```python
from build123d import *

# Parameters (mm, degrees)
SALIENTE_EXTRUIR1_DEPTH = 13.746
CROQUIS2_R              = 15.5
CORTAR_EXTRUIR1_DEPTH   = 10
CROQUIS3_R              = 1.6
CORTAR_EXTRUIR2_DEPTH   = 10
SALIENTE_EXTRUIR2_START = -4
CROQUIS4_R              = 1.5
SALIENTE_EXTRUIR2_DEPTH = 4
CORTAR_EXTRUIR3_DEPTH   = 45.978374576
CROQUIS6_R              = 1.5
CORTAR_EXTRUIR4_DEPTH   = 44.749194214
CROQUIS7_R              = 2.05
CORTAR_EXTRUIR5_DEPTH   = 6
CROQUIS8_R              = 4
CORTAR_EXTRUIR6_DEPTH   = 0.746


# Read off the part's stored shape, not the designer's step: Saliente-Extruir1
with BuildPart() as part:
    # Saliente-Extruir1 outline → Saliente-Extruir1 (new body)
    with BuildSketch(Plane(origin=(0, 0, 0), x_dir=(1, 0, 0), z_dir=(0, 1, 0))):
        with BuildLine():
            Line((26.09194434, -20.692720824), (18.78711178, 5.224407236))
            ThreePointArc((18.78711178, 5.224407236), (-5.766161796, 18.627973001), (-18.453215474, -6.30308168))
            Line((-18.453215474, -6.30308168), (-12.857048648, -22.686698065))
            Line((-12.857048648, -22.686698065), (26.09194434, -20.692720824))
        make_face()
    extrude(amount=SALIENTE_EXTRUIR1_DEPTH)

    # Croquis2 → Cortar-Extruir1 (cut)
    with BuildSketch(Plane(origin=(0, 13.746, 0), x_dir=(1, 0, 0), z_dir=(0, 1, 0))):
        with Locations(Location((0, 0, 0), (0, 0, 270))):
            Circle(CROQUIS2_R)
    extrude(amount=-CORTAR_EXTRUIR1_DEPTH, mode=Mode.SUBTRACT)

    # Croquis3 → Cortar-Extruir2 (cut)
    with BuildSketch(Plane(origin=(0, 3.746, 0), x_dir=(1, 0, 0), z_dir=(0, 1, 0))):
        with Locations(Location((0, 0, 0), (0, 0, 270))):
            Circle(CROQUIS3_R)
    extrude(amount=-CORTAR_EXTRUIR2_DEPTH, mode=Mode.SUBTRACT)

    # Croquis4 → Saliente-Extruir2 (add)
    # profile 1 of 3: a face of its own
    with BuildSketch(Plane(origin=(0, 13.746, 0), x_dir=(1, 0, 0), z_dir=(0, 1, 0)).offset(SALIENTE_EXTRUIR2_START)):
        with BuildLine():
            Line((-17.399016653, -21.764305721), (-13.613741684, -20.471365889))
            Line((-13.613741684, -20.471365889), (-16.199621348, -12.900815951))
            Line((-16.199621348, -12.900815951), (-19.984896317, -14.193755782))
            ThreePointArc((-19.984896317, -14.193755782), (-22.477231454, -19.271970583), (-17.399016653, -21.764305721))
        make_face()
        with Locations(Location((-18.691956485, -17.979030752, 0), (0, 0, 270))):
            Circle(CROQUIS4_R, mode=Mode.SUBTRACT)
    # profile 2 of 3: a face of its own
    with BuildSketch(Plane(origin=(0, 13.746, 0), x_dir=(1, 0, 0), z_dir=(0, 1, 0)).offset(SALIENTE_EXTRUIR2_START)):
        with BuildLine():
            Line((23.921673943, -12.992725603), (26.09194434, -20.692720824))
            Line((26.09194434, -20.692720824), (29.941941951, -19.607585626))
            ThreePointArc((29.941941951, -19.607585626), (32.75563819, -14.658688833), (27.771671554, -11.907590405))
            Line((27.771671554, -11.907590405), (23.921673943, -12.992725603))
        make_face()
    # profile 3 of 3: a face of its own
    with BuildSketch(Plane(origin=(0, 13.746, 0), x_dir=(1, 0, 0), z_dir=(0, 1, 0)).offset(SALIENTE_EXTRUIR2_START)):
        with BuildLine():
            Line((-2.321, 23.759), (-2.321, 19.361378024))
            ThreePointArc((-2.321, 19.361378024), (1.699637522, 19.425787816), (5.648, 18.664139305))
            Line((5.648, 18.664139305), (5.648, 23.062))
            ThreePointArc((5.648, 23.062), (2.012, 27.395), (-2.321, 23.759))
        make_face()
        with Locations(Location((1.6635, 23.4105, 0), (0, 0, 270))):
            Circle(CROQUIS4_R, mode=Mode.SUBTRACT)
    extrude(amount=SALIENTE_EXTRUIR2_DEPTH)

    # Croquis5 → Cortar-Extruir3 (cut, through all)
    with BuildSketch(Plane(origin=(0, 13.746, 0), x_dir=(1, 0, 0), z_dir=(0, 1, 0))):
        with BuildLine():
            Line((25.521809268, -10.120190748), (26.141320794, -12.367178003))
            ThreePointArc((26.141320794, -12.367178003), (31.060606452, -15.160138551), (28.267645904, -20.079424208))
            Line((28.267645904, -20.079424208), (28.88715743, -22.326411463))
            ThreePointArc((28.88715743, -22.326411463), (33.307593706, -14.540627024), (25.521809268, -10.120190748))
        make_face()
    extrude(amount=-CORTAR_EXTRUIR3_DEPTH, mode=Mode.SUBTRACT)

    # Croquis6 → Cortar-Extruir4 (cut, through all)
    with BuildSketch(Plane(origin=(0, 13.746, 0), x_dir=(1, 0, 0), z_dir=(0, 1, 0))):
        with Locations(Location((27.204483349, -16.223301105, 0), (0, 0, 270))):
            Circle(CROQUIS6_R)
    extrude(amount=-CORTAR_EXTRUIR4_DEPTH, mode=Mode.SUBTRACT)

    # Croquis7 → Cortar-Extruir5 (cut)
    with BuildSketch(Plane.XZ):
        with Locations(Location((7.549608222, 17.636749548, 0), (0, 0, 270))):
            Circle(CROQUIS7_R)
    extrude(amount=-CORTAR_EXTRUIR5_DEPTH, mode=Mode.SUBTRACT)

    # Croquis8 → Cortar-Extruir6 (cut)
    with BuildSketch(Plane.XZ):
        with Locations(Location((0, 0, 0), (0, 0, 270))):
            Circle(CROQUIS8_R)
    extrude(amount=-CORTAR_EXTRUIR6_DEPTH, mode=Mode.SUBTRACT)


solid = part.part
```
Geometry: final body of the model. Coordinates: model frame, mm. A direction names the side the tool comes from. Give positions to 0.01 mm unless a question says otherwise; leave off trailing zeros. Write each loop counter-clockwise with the first axis right and the second up, starting at its lowest first coordinate (ties: lowest second). Pieces come first, ordered by that corner, then holes.
1. Section query C-C, the plane z = 8.5. Return loops of the section in (x, y).
2. Draft query along X for faces 1 (the flat face through (5.648, 12, -21)), 2 (the cylindrical face through (-3.905, 0.368, 0.867)), 3 (the cylindrical face through (-5.35, 6.78, -18.75)). Return one class per face: released by +X, released by -X, zero draft, split by the parting line, or undercut.
3. Section query A-A, the plane y = 7. Return loops of the section in (x, z).
4. Section query D-D, the plane y = 2.25. Return loops of the section in (x, z).
5. Line query: probe 1 along Y at (x, z) = (-9, -7.5); probe 2 along Y at (x, z) = (-15.5, 18); probe 3 along X at (y, z) = (11.25, -13.5). Output: solid intervals per line, ascending.
6. Section query B-B, the plane z = 0. Return loops of the section in (x, y), then the cut area to 3 significant figures.
7. Reachability of faces 4 (the flat face through (-18.07, 11.72, 13.54)), 5 (the flat face through (29, 9.746, 16)), 6 (the flat face through (8, 6, 18)), 7 (the cylindrical face through (15.368, 8.816, -2.018)) from +Z, -Z, +X, -X, +Y, -Y: full face, straight path, thin tool, end or side. Return the list, or none.
8. Pin query (flat end, axial travel): P1, Ø25, axis at x = 0, z = 0, coming from the +Y side; P2, Ø2, axis at x = 14.5, y = 8, coming from the +Z side; P3, Ø3, axis at y = 11, z = -21, coming from the -X side. Return the tip coordinate at first contact, or that it passes through.
Computed:
1. outline: (-17.7, 0) - (22.66, 0) - (22.66, 13.75) - (12.96, 13.75) - (12.96, 3.75) - (-12.96, 3.75) - (-12.96, 13.75) - (-17.7, 13.75) - close
2. face 1: released by +X
2. face 2: undercut
2. face 3: split by the parting line
3. outline: (-18.45, 6.3) arc R19.5 ccw (long way) to (18.79, -5.22) - (26.09, 20.69) - (-12.86, 22.69) - close; hole circle Ø31 at (0, 0)
4. outline: (-18.45, 6.3) arc R19.5 ccw (long way) to (18.79, -5.22) - (26.09, 20.69) - (-12.86, 22.69) - close; hole circle Ø3.2 at (0, 0); hole circle Ø4.1 at (7.55, 17.64)
5. probe 1: y = 0 to 3.75
5. probe 2: y = 9.75 to 13.75
5. probe 3: x = -14.07 to -7.62, 7.62 to 14.07
6. outline: (-19.5, 0) - (-4, 0) - (-4, 0.75) - (-1.6, 0.75) - (-1.6, 3.75) - (-15.5, 3.75) - (-15.5, 13.75) - (-19.5, 13.75) - close; (1.6, 0.75) - (4, 0.75) - (4, 0) - (20.26, 0) - (20.26, 13.75) - (15.5, 13.75) - (15.5, 3.75) - (1.6, 3.75) - close
6. area: 221 mm2
7. face 4: -X, +Y, -Y
7. face 5: -Z, +X, -Y
7. face 6: -Y
7. face 7: +Y
8. P1: stops at y = 3.75
8. P2: stops at z = 21.34
8. P3: stops at x = -2.32
